from build123d import *

# Parameters (mm, degrees)
BOSS_EXTRUDE1_DEPTH      = 14
BOSS_EXTRUDE1_DEPTH_BACK = 14
SKETCH1_R                = 17.5
SKETCH3_R                = 10
CUT_EXTRUDE1_DEPTH       = 20
CUT_EXTRUDE3_DEPTH       = 39
SKETCH5_R                = 1.75
CUT_EXTRUDE4_DEPTH       = 39
SKETCH6_R                = 3.25
CUT_EXTRUDE5_DEPTH       = 1.5


with BuildPart() as part:
    # Sketch1 → Boss-Extrude1 (new, two sides: drawn at the far end of the back side and taken through both)
    with BuildSketch(Plane(origin=(0, 0, 0), x_dir=(1, 0, 0), z_dir=(0, 1, 0)).offset(-BOSS_EXTRUDE1_DEPTH_BACK)):
        Circle(SKETCH1_R)
        with BuildLine():
            Line((20, 17.5), (0, 17.5))
            ThreePointArc((0, 17.5), (12.374368671, 12.374368671), (17.5, 0))
            ThreePointArc((17.5, 0), (12.37436868, -12.374368661), (2.7e-08, -17.5))
            Line((2.7e-08, -17.5), (20, -17.5))
            Line((20, -17.5), (20, 17.5))
        make_face()
    extrude(amount=BOSS_EXTRUDE1_DEPTH + BOSS_EXTRUDE1_DEPTH_BACK)

    # Sketch3 → Cut-Extrude1 (cut)
    with BuildSketch(Plane(origin=(20, 0, 0), x_dir=(0, 0, -1), z_dir=(1, 0, 0))):
        Circle(SKETCH3_R)
    extrude(amount=-CUT_EXTRUDE1_DEPTH, mode=Mode.SUBTRACT)

    # Sketch4 → Cut-Extrude3 (cut)
    with BuildSketch(Plane(origin=(20, 0, 0), x_dir=(0, 0, -1), z_dir=(1, 0, 0))):
        Polygon((-29.488337181, 0), (29.963955523, 0), (3.938373511, 60.173176489), align=None)
    extrude(amount=-CUT_EXTRUDE3_DEPTH, mode=Mode.SUBTRACT)

    # Sketch5 → Cut-Extrude4 (cut)
    with BuildSketch(Plane(origin=(0, 0, 0), x_dir=(1, 0, 0), z_dir=(0, 1, 0))):
        with Locations(Location((15, 13.75, 0), (0, 0, 270))):
            Circle(SKETCH5_R)
        with Locations(Location((6, 13.75, 0), (0, 0, 270))):
            Circle(SKETCH5_R)
        with Locations(Location((-3, 13.75, 0), (0, 0, 270))):
            Circle(SKETCH5_R)
        with Locations(Location((-3, 0, 0), (0, 0, 270))):
            Circle(SKETCH5_R)
        with Locations(Location((-12, 0, 0), (0, 0, 270))):
            Circle(SKETCH5_R)
        with Locations(Location((15, -13.75, 0), (0, 0, 270))):
            Circle(SKETCH5_R)
        with Locations(Location((6, -13.75, 0), (0, 0, 270))):
            Circle(SKETCH5_R)
        with Locations(Location((-3, -13.75, 0), (0, 0, 270))):
            Circle(SKETCH5_R)
    extrude(amount=-CUT_EXTRUDE4_DEPTH, mode=Mode.SUBTRACT)

    # Sketch6 → Cut-Extrude5 (cut)
    with BuildSketch(Plane.XZ.offset(14)):
        with Locations(Location((-3, 13.75, 0), (0, 0, 270))):
            Circle(SKETCH6_R)
        with Locations(Location((6, 13.75, 0), (0, 0, 270))):
            Circle(SKETCH6_R)
        with Locations(Location((15, 13.75, 0), (0, 0, 270))):
            Circle(SKETCH6_R)
        with Locations(Location((-12, 0, 0), (0, 0, 270))):
            Circle(SKETCH6_R)
        with Locations(Location((-3, 0, 0), (0, 0, 270))):
            Circle(SKETCH6_R)
        with Locations(Location((-3, -13.75, 0), (0, 0, 270))):
            Circle(SKETCH6_R)
        with Locations(Location((6, -13.75, 0), (0, 0, 270))):
            Circle(SKETCH6_R)
        with Locations(Location((15, -13.75, 0), (0, 0, 270))):
            Circle(SKETCH6_R)
    extrude(amount=-CUT_EXTRUDE5_DEPTH, mode=Mode.SUBTRACT)


solid = part.part
Work out the finished part from the listing and answer in its coordinate system (mm). A direction names the side the tool comes from. Round coordinates to 2 decimals unless told otherwise and drop trailing zeros. Write each loop counter-clockwise with the first axis right and the second up, starting at its lowest first coordinate (ties: lowest second). Pieces come first, ordered by that corner, then holes. Notation, with made-up numbers: (65.5, 44.5) - (99.5, 44.5) arc R21 ccw to (99.5, 58.5) - close; hole circle Ø6 at (-14, -2). An arc over 180 degrees is marked (long way). Answer in a Markdown table with one row per item. Add a question column.
1. A cutting plane is placed at B-B, the plane z = -13.75. Determine the outline of the cut face in (x, y).
2. A cutting plane is placed at D-D, the plane x = 10. Determine the outline of the cut face in (y, z).
3. The mould has two halves that part along X. Classify faces 1 (the flat face through (1, -14, 0)), 2 (the flat face through (0, -4, 0)), 3 (the flat face through (13.6, -12.5, -15.1)): +X half, -X half, draft (parallel to the pull), parting line (faces both ways), or undercut.
4. Given pin 1 (4 mm diameter, centred on x = -3, z = -13.75, fed in from +Y); pin 2 (4 mm diameter, centred on x = -12, z = 0, fed in from -Y); pin 3 (2 mm diameter, centred on x = -3, z = 0, fed in from -Y); pin 4 (2 mm diameter, centred on y = -11.5, z = 4, fed in from -X), each flat-ended and moving along its own axis, determine where each tip first touches the part or whether it passes through.
5. A cutting plane is placed at C-C, the plane z = 0. Determine the outline of the cut face in (x, y).
6. Find the intervals of material crossed by line 1 along X through (y, z) = (-13.05, 0); line 2 along X through (y, z) = (-3.75, -13.75); line 3 along X through (y, z) = (-1.5, -13.5), in increasing order. Write a range as from..to.
7. For faces 4 (the cylindrical face through (10, -10, 0)), 5 (the cylindrical face through (-3.67, -6.162, -12.133)), 6 (the cylindrical face through (18.222, -13.26, 14.173)), determine the directions among +Z, -Z, +X, -X, +Y, -Y from which every point of the face is accessible in a straight line to the end or side of a thin tool.
8. A cutting plane is placed at A-A, the plane x = 6. Determine the outline of the cut face in (y, z).
Worked out:
| question | item | result |
|---|---|---|
| 1 | outline | (-10.83, -14) - (-6.25, -14) - (-6.25, -12.5) - (-4.75, -12.5) - (-4.75, 0) - (-10.83, 0) - close; (-1.25, -12.5) - (0.25, -12.5) - (0.25, -14) - (2.75, -14) - (2.75, -12.5) - (4.25, -12.5) - (4.25, 0) - (-1.25, 0) - close; (7.75, -12.5) - (9.25, -12.5) - (9.25, -14) - (11.75, -14) - (11.75, -12.5) - (13.25, -12.5) - (13.25, 0) - (7.75, 0) - close; (16.75, -12.5) - (18.25, -12.5) - (18.25, -14) - (20, -14) - (20, 0) - (16.75, 0) - close |
| 2 | outline | (-14, -17.5) - (0, -17.5) - (0, -10) arc R10 cw to (0, 10) - (0, 17.5) - (-14, 17.5) - close |
| 3 | face 1 | draft |
| 3 | face 2 | +X half |
| 3 | face 3 | undercut |
| 4 | pin 1 | y = 0 |
| 4 | pin 2 | y = -12.5 |
| 4 | pin 3 | through |
| 4 | pin 4 | x = -17.24 |
| 5 | outline | (-17.5, -14) - (-15.25, -14) - (-15.25, -12.5) - (-13.75, -12.5) - (-13.75, 0) - (-17.5, 0) - close; (-10.25, -12.5) - (-8.75, -12.5) - (-8.75, -14) - (-6.25, -14) - (-6.25, -12.5) - (-4.75, -12.5) - (-4.75, 0) - (-10.25, 0) - close; (-1.25, -12.5) - (0.25, -12.5) - (0.25, -14) - (20, -14) - (20, -10) - (0, -10) - (0, 0) - (-1.25, 0) - close |
| 6 | line 1 | -17.5..-15.25, -8.75..-6.25, 0.25..20 |
| 6 | line 2 | -10.83..-4.75, -1.25..4.25, 7.75..13.25, 16.75..20 |
| 6 | line 3 | -11.14..-4.73, -1.27..4.27, 7.73..13.27, 16.73..20 |
| 7 | face 4 | +X, +Y |
| 7 | face 5 | +Y, -Y |
| 7 | face 6 | -Y |
| 8 | outline | (-14, -17.5) - (0, -17.5) - (0, -15.5) - (-12.5, -15.5) - (-12.5, -17) - (-14, -17) - close; (-14, -10.5) - (-12.5, -10.5) - (-12.5, -12) - (0, -12) - (0, -10) arc R10 cw to (0, 10) - (0, 12) - (-12.5, 12) - (-12.5, 10.5) - (-14, 10.5) - close; (-14, 17) - (-12.5, 17) - (-12.5, 15.5) - (0, 15.5) - (0, 17.5) - (-14, 17.5) - close |
